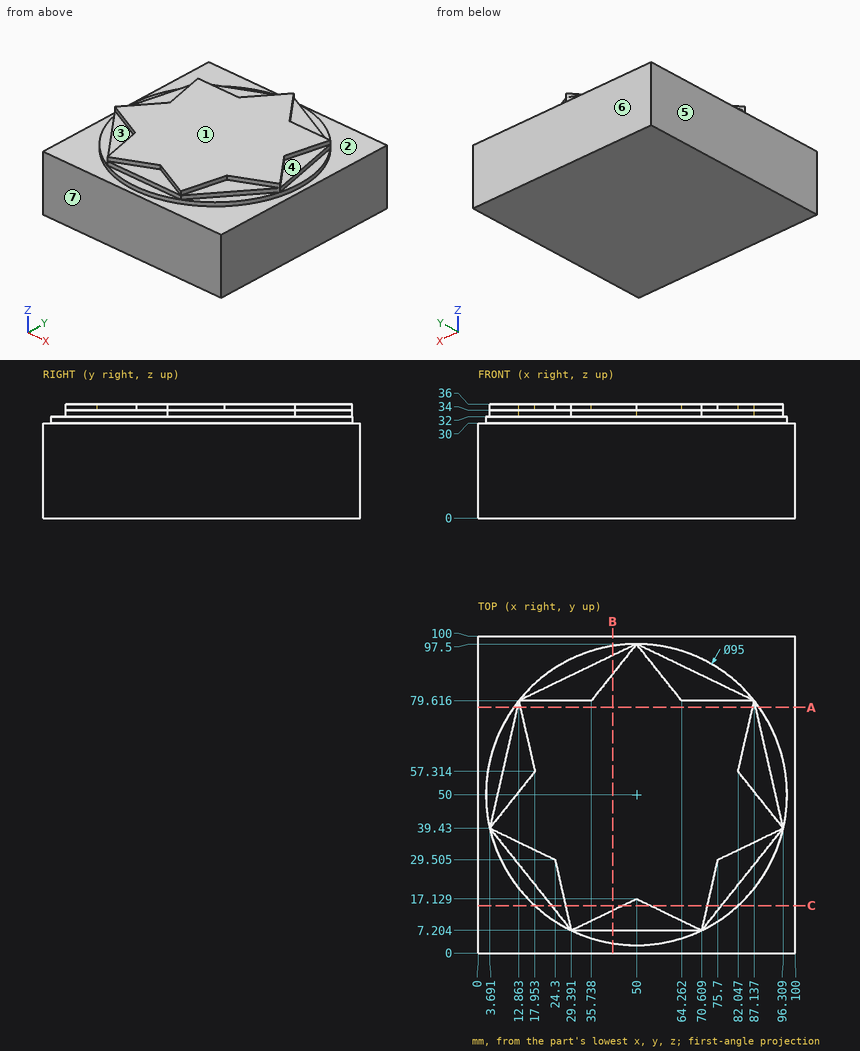
Geometry check sheet. Reference: drawing and pictorial views, mm from the part's lowest x, y, z. A direction names the side the tool comes from. Give positions to 0.01 mm unless a question says otherwise; leave off trailing zeros. Order: outer loops, then holes, each group sorted by start corner. A loop starts at its lowest first (then second) coordinate and runs counter-clockwise, first axis right, second up. Notation, with made-up numbers: M -33,74.5 L 6,74.5 A26 ccw 6,100.5 Z; hole C -9.75,-35.5 d3. An arc over 180 degrees is marked long. Return JSON: item names as keys, results as strings. Group by question number.
1) Access from +Z, -Z, +X, -X, +Y, -Y to the whole of each face (thin tool, end or side, straight path). Record for the marked faces 1, 2 and 3.
2) Mould release check, pull along Y, two halves, no side actions. Record for the marked faces 4, 5, 6 and 7: pulls with the +Y half, pulls with the -Y half, needs draft (parallel to the pull), parting line crosses it, or undercut.
3) Go/stop test with flat-tipped pins: pin 1 Ø4 at (x, y) = (50, 4) entering from +Z; pin 2 Ø4.5 at (x, y) = (8.5, 65) entering from +Z; pin 3 Ø1.6 at (x, z) = (19, 35) entering from +Y. Record where each tip stops, or that it passes through.
4) Section check B-B on x = 42.5. Record the cut outline in (y, z) (1 decimal), and give its area (3 significant figures).
5) Scan lines: line 1 (Z direction, x = 5.5, y = 74.5); line 2 (Z direction, x = 80, y = 29); line 3 (Y direction, x = 37.5, z = 32.5) (1 decimal). Record each from-to range of solid material in increasing order.
6) Section check A-A on y = 77.5. Record the cut outline in (x, z) (1 decimal), and give its area (3 significant figures).
7) Section check C-C on y = 15. Record the cut outline in (x, z).
Answer block:
{
 "1": {"face 1": "+Z, +X, -X, +Y, -Y", "face 2": "+Z", "face 3": "+Z, -X, -Y"},
 "2": {"face 4": "undercut", "face 5": "needs draft", "face 6": "pulls with the +Y half", "face 7": "pulls with the -Y half"},
 "3": {"pin 1": "stops at z = 32", "pin 2": "stops at z = 34", "pin 3": "stops at y = 79.62"},
 "4": {"outline": "M 0,0 L 100,0 L 100,30 L 96.9,30 L 96.9,32 L 93.9,32 L 93.9,34 L 88.1,34 L 88.1,36 L 13.5,36 L 13.5,34 L 7.2,34 L 7.2,32 L 3.1,32 L 3.1,30 L 0,30 Z", "area": "3,510 mm^2"},
 "5": {"line 1": "z = 0 to 30", "line 2": "z = 0 to 34", "line 3": "y = 7.2 to 91.5"},
 "6": {"outline": "M 0,0 L 100,0 L 100,30 L 88.7,30 L 88.7,32 L 87.6,32 L 87.6,34 L 86.7,34 L 86.7,36 L 13.3,36 L 13.3,34 L 12.4,34 L 12.4,32 L 11.3,32 L 11.3,30 L 0,30 Z", "area": "3,450 mm^2"},
 "7": {"outline": "M 0,0 L 100,0 L 100,30 L 82.11,30 L 82.11,32 L 76.83,32 L 76.83,34 L 72.39,34 L 72.39,36 L 54.42,36 L 54.42,34 L 45.58,34 L 45.58,36 L 27.61,36 L 27.61,34 L 23.17,34 L 23.17,32 L 17.89,32 L 17.89,30 L 0,30 Z"}
}
